Source: CAD feature listing. Evaluate the final solid. Frame: model axes, mm. A direction names the side the tool comes from. Round coordinates to 2 decimals unless told otherwise and drop trailing zeros. Order: outer loops, then holes, each group sorted by start corner. A loop starts at its lowest first (then second) coordinate and runs counter-clockwise, first axis right, second up. Notation, with made-up numbers: (88, 89.5) - (138, 89.5) arc R26 cw to (138, 103.5) - close; hole circle Ø1 at (-37, 89.5). An arc over 180 degrees is marked (long way). Put each result on its own line as item: value. Start each with the question number.
1) Section D-D on z = -14. Output: boundary loops of the cut face in (x, y), then the cut area to 3 significant figures.
2) Section B-B on x = -111. Output: boundary loops of the cut face in (y, z).
3) Access query for faces 1 (the face through (-86.786, 10, -19)), 2 (the face through (-107, 25, -19.977)), 3 (the face through (-116.786, 11, -15)), 4 (the face through (-96.786, 25, -25)), 5 (the face through (-97, 15, -9.977)). Directions: +Z, -Z, +X, -X, +Y, -Y. A direction counts if a zero-diameter tool reaches every point of the face in a straight line with its end or side. Return the directions, or none.
4) Section C-C on x = -102. Output: boundary loops of the cut face in (y, z), then the cut area to 3 significant figures.
5) Contact query for flat-ended pins moving along their axis: P1, Ø3, axis at x = -95, y = 14.5, coming from the +Z side; P2, Ø8, axis at x = -92, z = -7, coming from the +Y side; P3, Ø1, axis at y = 24.5, z = -25.5, coming from the +X side. Output: stop coordinate, or through.
6) Line query: probe 1 along X at (y, z) = (26.5, -20.5); probe 2 along Y at (x, z) = (-88.5, -26); probe 3 along Z at (x, y) = (-106, 16.75). Output: solid intervals per line, ascending. Write a range as [from, to].
7) Section A-A on z = -25. Output: boundary loops of the cut face in (x, y).
```python
from build123d import *

# Parameters (mm, degrees)
CROQUIS1_W              = 30
CROQUIS1_H              = 30
SALIENTE_EXTRUIR1_DEPTH = 10
SALIENTE_EXTRUIR2_DEPTH = 10
CROQUIS5_W              = 20
CROQUIS5_H              = 10
SALIENTE_EXTRUIR3_DEPTH = 10


with BuildPart() as part:
    # Croquis1 → Saliente-Extruir1 (new body)
    with BuildSketch(Plane(origin=(0, 0, 0), x_dir=(1, 0, 0), z_dir=(0, 1, 0))):
        with Locations((-101.786127258, 14.977187745)):
            Rectangle(CROQUIS1_W, CROQUIS1_H)
    extrude(amount=SALIENTE_EXTRUIR1_DEPTH)

    # Croquis3 → Saliente-Extruir2 (add)
    with BuildSketch(Plane(origin=(0, 10, 0), x_dir=(1, 0, 0), z_dir=(0, 1, 0))):
        Polygon((-116.786127258, 29.977187745), (-106.786127258, 29.977187745), (-86.786127258, 29.977187745), (-86.786127258, 9.977187745), (-106.786127258, 9.977187745), (-106.786127258, -0.022812255), (-116.786127258, -0.022812255), align=None)
    extrude(amount=SALIENTE_EXTRUIR2_DEPTH)

    # Croquis5 → Saliente-Extruir3 (add)
    with BuildSketch(Plane(origin=(0, 20, 0), x_dir=(1, 0, 0), z_dir=(0, 1, 0))):
        with Locations((-106.786127258, 24.977187745)):
            Rectangle(CROQUIS5_W, CROQUIS5_H)
    extrude(amount=SALIENTE_EXTRUIR3_DEPTH)


solid = part.part
```
Answer sheet:
1. outline: (-116.79, 0) - (-86.79, 0) - (-86.79, 20) - (-116.79, 20) - close
1. area: 600 mm^2
2. outline: (0, -29.98) - (30, -29.98) - (30, -19.98) - (20, -19.98) - (20, 0.02) - (0, 0.02) - close
3. face 1: +Z, -Z, +X, +Y, -Y
3. face 2: +Z, +X, -X, +Y
3. face 3: +Z, -Z, -X, +Y, -Y
3. face 4: +Z, -Z, +X, +Y
3. face 5: +Z, +X, +Y
4. outline: (0, -29.98) - (30, -29.98) - (30, -19.98) - (20, -19.98) - (20, -9.98) - (10, -9.98) - (10, 0.02) - (0, 0.02) - close
4. area: 600 mm^2
5. P1: z = -9.98
5. P2: y = 20
5. P3: x = -96.79
6. probe 1: [-116.79, -96.79]
6. probe 2: [0, 20]
6. probe 3: [-29.98, -9.98]
7. outline: (-116.79, 0) - (-86.79, 0) - (-86.79, 20) - (-96.79, 20) - (-96.79, 30) - (-116.79, 30) - close
